Can you work these out from the model? Positions are in its coordinate system, mm. Round coordinates to 2 decimals unless told otherwise and drop trailing zeros. Order: outer loops, then holes, each group sorted by start corner. A loop starts at its lowest first (then second) coordinate and runs counter-clockwise, first axis right, second up. Notation, with made-up numbers: M -22,-29.75 L 13,-29.75 A15 cw 13,-4.75 Z; hole C 55.25,80.25 d3. An arc over 180 degrees is marked long. One line per question, with ' | ' between items.
```python
from build123d import *

# Parameters (mm, degrees)
F1_DEPTH = 25
F2_R     = 5


with BuildPart() as f1:
    # F0 (on Front) → F1 (new body)
    with BuildSketch(Plane.XZ):
        Polygon((18.595429, -51.854381), (47.576278, -27.769849), (54.295658, 9.308504), (35.609496, 42.031304), (0.261255, 55.08719), (-35.20923, 42.367167), (-54.204925, 9.823076), (-47.837534, -27.317341), (-19.086428, -51.675671), align=None)
    extrude(amount=F1_DEPTH)

    # F2
    f2_edges = [f1.edges().sort_by_distance(p)[0] for p in [
        (33.085854, -25, -39.812115),
        (50.935968, -25, -9.230672),
        (44.952577, -25, 25.669904),
        (17.935376, -25, 48.559247),
        (-17.473987, -25, 48.727179),
        (-44.707078, -25, 26.095122),
        (-51.02123, -25, -8.747133),
        (-33.461981, -25, -39.496506),
        (-0.2455, -25, -51.765026),
    ]]
    fillet(f2_edges, radius=F2_R)


solid = f1.part
```
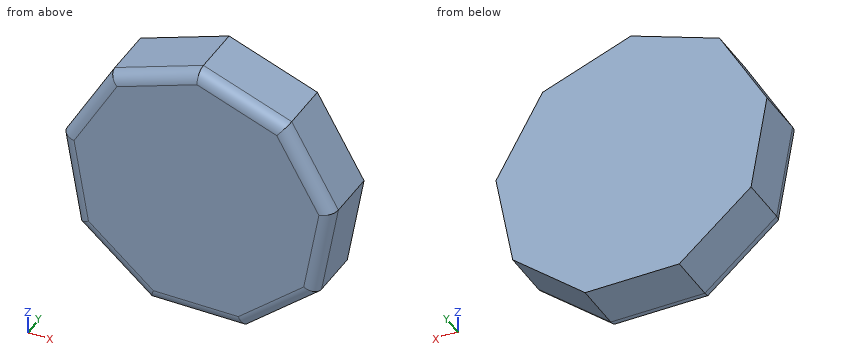
(1) Please list where these lines run through material, in increasing order: probe 1 along Z at (x, y) = (-16, -13.25); probe 2 along Z at (x, y) = (22.5, -16); probe 3 along X at (y, z) = (-12.5, -29). Write a range as [from, to].
Final values:
probe 1: [-51.69, 49.26] | probe 2: [-48.61, 46.87] | probe 3: [-45.85, 46.1]
(2) If we section it at B-B on y = -22.75: Please give me the cut outline in (x, z).
Final values:
outline: M -53.34,9.67 L -47.08,-26.88 L -18.78,-50.85 L 18.3,-51.03 L 46.82,-27.33 L 53.43,9.16 L 35.04,41.36 L 0.26,54.21 L -34.65,41.69 Z
(3) If we section it at A-A on y = -15: Please give me the cut outline in (x, z), plus the area to 3 significant figures.
Final values:
outline: M -54.2,9.82 L -47.84,-27.32 L -19.09,-51.68 L 18.6,-51.85 L 47.58,-27.77 L 54.3,9.31 L 35.61,42.03 L 0.26,55.09 L -35.21,42.37 Z | area: 8,780 mm^2
(4) Will these pins go through, and if not, where does the flat tip stop? pin 1 Ø4 at (x, y) = (-6.5, -22) entering from -Z; pin 2 Ø12 at (x, z) = (21, 7) entering from +Y; pin 3 Ø6 at (x, y) = (14, -20) entering from +Z; pin 4 Ø4 at (x, y) = (7, -17.5) entering from -Z.
Final values:
pin 1: z = -51.74 | pin 2: y = 0 | pin 3: z = 51.12 | pin 4: z = -51.81
